from build123d import *

# Parameters (mm, degrees)
F1_DEPTH    = 50.8
F2_W        = 57.15
F2_H        = 38.1
F3_DEPTH    = 6.35
F4_W        = 23.114
F4_H        = 6.604
F4_W_2      = 0.9801145643
F4_H_2      = 5.08
F5_DEPTH    = 2.54
F4_R        = 2.667
F6_DEPTH    = 1.27
F8_DEPTH    = 0.8001
F9_T1_DEPTH = 71.4372925246
F9_T3_DEPTH = 69.6542925277
F11_DEPTH   = 0.8001
F13_DEPTH   = 0.8001
F15_DEPTH   = 0.254
F16_W       = 18.161
F16_H       = 19.05
F17_DEPTH   = 0.8001
F18_DEPTH   = 50.8
F19_W       = 127
F19_H       = 25.4
F20_DEPTH   = 12.7
F21_DEPTH   = 5.08
F22_R       = 1.397
F23_R       = 1.397
F24_DEPTH   = 25.4


# Not quite as in the source:
# - a fillet or chamfer that OpenCascade refuses, or shapes differently, is made with other operations: its cross-section is extruded or revolved along the edge and cut away or added


with BuildPart() as f1:
    # F0 (on Front) → F1 (new body)
    with BuildSketch(Plane.XZ):
        with BuildLine():
            Line((-68.745650351, 20.2095657587), (-68.745650351, 0))
            Line((-68.745650351, 0), (-55.97953596, 0))
            ThreePointArc((-55.97953596, 0), (-44.54953596, 11.43), (-33.11953596, 0))
            Line((-33.11953596, 0), (44.1833575737, 0))
            ThreePointArc((44.1833575737, 0), (55.6133575737, 11.43), (67.0433575737, 0))
            Line((67.0433575737, 0), (83.654349649, 0))
            Line((83.654349649, 0), (83.654349649, 19.05))
            Line((83.654349649, 19.05), (20.154349649, 19.05))
            Line((20.154349649, 19.05), (20.154349649, 50.8))
            Line((20.154349649, 50.8), (-20.485650351, 50.8))
            Line((-20.485650351, 50.8), (-27.103371678, 28.9188353957))
            Line((-27.103371678, 28.9188353957), (-68.745650351, 20.2095657587))
        make_face()
        with BuildLine():
            ThreePointArc((-33.11953596, 0), (-44.54953596, 11.43), (-55.97953596, 0))
            Line((-55.97953596, 0), (-33.11953596, 0))
        make_face()
        with BuildLine():
            ThreePointArc((67.0433575737, 0), (55.6133575737, 11.43), (44.1833575737, 0))
            Line((44.1833575737, 0), (67.0433575737, 0))
        make_face()
    extrude(amount=F1_DEPTH)

    # F2 (on face) → F3 (cut)
    with BuildSketch(Plane.XY.offset(19.05)):
        with Locations((48.729349649, -25.4)):
            Rectangle(F2_W, F2_H)
    extrude(amount=-F3_DEPTH, mode=Mode.SUBTRACT)

    # F4 (on face) → F5 (join)
    with BuildSketch(Plane(origin=(-68.745650351, 0, 0), x_dir=(0, -1, 0), z_dir=(-1, 0, 0))):
        with Locations((25.4, 9.8053713022)):
            Rectangle(F4_W, F4_H)
        Polygon((36.195, 12.3453713022), (36.195, 7.2653713022), (32.6746520766, 7.2653713022), (31.6945375124, 7.2653713022), (29.2964520766, 7.2653713022), (28.3163375124, 7.2653713022), (25.9182520766, 7.2653713022), (24.9381375124, 7.2653713022), (22.5400520766, 7.2653713022), (21.5599375124, 7.2653713022), (19.1618520766, 7.2653713022), (18.1817375124, 7.2653713022), (14.605, 7.2653713022), (14.605, 12.3453713022), (18.1817375124, 12.3453713022), (19.1618520766, 12.3453713022), (21.5599375124, 12.3453713022), (22.5400520766, 12.3453713022), (24.9381375124, 12.3453713022), (25.9182520766, 12.3453713022), (28.3163375124, 12.3453713022), (29.2964520766, 12.3453713022), (31.6945375124, 12.3453713022), (32.6746520766, 12.3453713022), align=None, mode=Mode.SUBTRACT)
        with Locations((18.6717947945, 9.8053713022)):
            Rectangle(F4_W_2, F4_H_2)
        with Locations((22.0499947945, 9.8053713022)):
            Rectangle(F4_W_2, F4_H_2)
        with Locations((25.4281947945, 9.8053713022)):
            Rectangle(F4_W_2, F4_H_2)
        with Locations((28.8063947945, 9.8053713022)):
            Rectangle(F4_W_2, F4_H_2)
        with Locations((32.1845947945, 9.8053713022)):
            Rectangle(F4_W_2, F4_H_2)
    extrude(amount=F5_DEPTH)

    # F4 (on face) → F6 (join)
    with BuildSketch(Plane(origin=(-68.745650351, 0, 0), x_dir=(0, -1, 0), z_dir=(-1, 0, 0))):
        with Locations((6.35, 9.8351975903)):
            Circle(F4_R)
        with Locations((44.45, 9.8351975903)):
            Circle(F4_R)
    extrude(amount=F6_DEPTH)

    # F7 (on face) → F8 (cut)
    with BuildSketch(Plane(origin=(-32.8452255156, 0, 9.9336828416), x_dir=(0, -1, 0), z_dir=(-0.9571813038, 0, 0.2894891219))):
        Polygon((33.562220633, 22.6956736296), (47.9775152107, 22.6956736296), (47.9775152107, 40.2216736296), (2.2575152107, 40.2216736296), (2.2575152107, 22.6956736296), (16.4677330811, 22.6956736296), (15.0759897713, 29.1358400136), (13.6842464615, 33.1220440567), (16.4677330811, 29.1358400136), (17.814220633, 22.6956736296), (32.2157330811, 22.6956736296), (30.8239897713, 29.1358400136), (29.4322464615, 33.1220440567), (32.2157330811, 29.1358400136), align=None)
    extrude(amount=-F8_DEPTH, mode=Mode.SUBTRACT)

    # F9: fillet of radius 5.08 on 2 edges, made by hand

    # F9_s2 → F9_t1 (cut)
    with BuildSketch(Plane.XZ.offset(-10.3186462623)):
        with BuildLine():
            ThreePointArc((-64.7056051643, 21.0545205498), (-67.6083252331, 19.2854983904), (-68.745650351, 16.0821072538))
            Line((-68.745650351, 16.0821072538), (-68.745650351, 20.2095657587))
            Line((-68.745650351, 20.2095657587), (-64.7056051643, 21.0545205498))
        make_face()
    extrude(amount=F9_T1_DEPTH, mode=Mode.SUBTRACT)

    # F9_s4 → F9_t3 (cut)
    with BuildSketch(Plane.XZ.offset(-9.4271462638)):
        with BuildLine():
            ThreePointArc((-21.5772728687, 47.1906047393), (-19.74263992, 49.7990361653), (-16.7147918455, 50.8))
            Line((-16.7147918455, 50.8), (-20.485650351, 50.8))
            Line((-20.485650351, 50.8), (-21.5772728687, 47.1906047393))
        make_face()
    extrude(amount=F9_T3_DEPTH, mode=Mode.SUBTRACT)

    # F10 (on face) → F11 (join)
    with BuildSketch(Plane.XZ.offset(50.8)):
        Polygon((13.9938081476, 45.7206499122), (-16.7147918455, 45.72), (-21.5772728687, 29.6424496777), (-21.5772728687, 5.5124496777), (13.9827271313, 5.5124514391), align=None)
    extrude(amount=F11_DEPTH)

    # F12 (on face) → F13 (join)
    with BuildSketch(Plane(origin=(0, 0, 0), x_dir=(-1, 0, 0), z_dir=(0, 1, 0))):
        Polygon((21.566192252, 29.6467966337), (16.7147918455, 45.72), (-13.993807748, 45.7249966337), (-13.993807748, 5.5167966337), (21.566192252, 5.5167966337), align=None)
    extrude(amount=F13_DEPTH)

    # F14 (on face) → F15 (join)
    with BuildSketch(Plane(origin=(0, 0.8001, 0), x_dir=(-1, 0, 0), z_dir=(0, 1, 0))):
        Polygon((-11.5635488182, 29.6467966337), (18.8161898404, 29.6467966337), (14.9059221148, 43.1567057967), (-11.5635488182, 43.1567057967), align=None)
    extrude(amount=-F15_DEPTH)

    # F16 (on face) → F17 (cut)
    with BuildSketch(Plane.YZ.offset(20.154349649)):
        with Locations((-35.3695, 38.1)):
            Rectangle(F16_W, F16_H)
        with Locations((-15.4305, 38.1)):
            Rectangle(F16_W, F16_H)
    extrude(amount=-F17_DEPTH, mode=Mode.SUBTRACT)

    # F0 (on Front) → F18 (cut)
    with BuildSketch(Plane.XZ):
        with BuildLine():
            ThreePointArc((67.0433575737, 0), (55.6133575737, 11.43), (44.1833575737, 0))
            Line((44.1833575737, 0), (67.0433575737, 0))
        make_face()
        with BuildLine():
            ThreePointArc((-33.11953596, 0), (-44.54953596, 11.43), (-55.97953596, 0))
            Line((-55.97953596, 0), (-33.11953596, 0))
        make_face()
    extrude(amount=F18_DEPTH, mode=Mode.SUBTRACT)

    # F19 (on face) → F20 (join)
    with BuildSketch(Plane(origin=(0, 0, 0), x_dir=(1, 0, 0), z_dir=(0, 0, -1))):
        with Locations((6.3173042834, 25.4)):
            Rectangle(F19_W, F19_H)
    extrude(amount=-F20_DEPTH)

    # F21 (add): a face of the model
    f21_faces = [f1.faces().sort_by_distance(p)[0] for p in [
        (7.7936035623, -25.4, 0),
    ]]
    extrude(f21_faces, amount=F21_DEPTH)

    # F22 (on face) + F23 (on face) → F24 (cut)
    with BuildSketch(Plane(origin=(0, -12.7, 0), x_dir=(-1, 0, 0), z_dir=(0, 1, 0))):
        with Locations((-55.6133575737, 0)):
            Circle(F22_R)
    with BuildSketch(Plane(origin=(0, -12.7, 0), x_dir=(-1, 0, 0), z_dir=(0, 1, 0))):
        with Locations((44.54953596, 0)):
            Circle(F23_R)
    extrude(amount=-F24_DEPTH, mode=Mode.SUBTRACT)


solid = f1.part
Design review of the part built by this model. Coordinates are the model's own, in mm. A direction names the side the tool comes from. Round coordinates to 2 decimals unless told otherwise and drop trailing zeros. Write each loop counter-clockwise with the first axis right and the second up, starting at its lowest first coordinate (ties: lowest second). Pieces come first, ordered by that corner, then holes. Notation, with made-up numbers: (33.25, 24.25) -> (76.25, 24.25) arc R30 ccw to (76.25, 55.25) -> close; hole circle Ø10 at (35.5, 77.25). An arc over 180 degrees is marked (long way). One line per item, written item: value. Start each with the question number.
Q1. Add section A-A (x = -41). Give the boundary of the cut face in (y, z), then the cut area to 3 significant figures.
Q2. To check wall thickness, follow probe 1 along X at (y, z) = (-28.5, 1); probe 2 along X at (y, z) = (-8.5, 6); probe 3 along Z at (x, y) = (62.5, -20). State the ranges of each line that lie inside material, in increasing order.
Q3. Insertion check: P1, Ø5, axis at y = -11.5, z = 23, coming from the -X side; P2, Ø1.5, axis at x = 50, y = -28, coming from the +Z side; P3, Ø5, axis at x = -46, z = 0, coming from the -Y side. Each pin has a flat end and moves straight along its axis. Give the tip position at first contact, or say it passes through.
Q4. Tool access review of faces 5 (the face through (48, -6.35, 16)), 6 (the face through (-43.154, -25.222, 0.061)), 7 (the face through (-33.12, -6, -3)), 8 (the face through (-45, -38.1, 3)), 9 (the face through (-69.37, -7.58, 7.47)): name each direction out of +Z, -Z, +X, -X, +Y, -Y from which nothing blocks a thin tool from reaching the whole face with its end or side.
Q5. The part is to be moulded in two halves that separate along X. For faces 1 (the face through (20.154, -25, 31)), 2 (the face through (-19.174, 0.394, 37.571)), 3 (the face through (-55.98, -6, -3)), 4 (the face through (6, 0, 5)), say which applies: pulls with the +X half, pulls with the -X half, needs draft (parallel to the pull), parting line crosses it, or undercut.
Response:
1. outline: (-50.8, 10.86) -> (-38.1, 10.86) -> (-38.1, -5.08) -> (-12.7, -5.08) -> (-12.7, 10.86) -> (0, 10.86) -> (0, 26.01) -> (-50.8, 26.01) -> close
1. area: 1,170 mm^2
2. probe 1: x = -68.75 to -45.53, -43.57 to 54.64, 56.59 to 83.65
2. probe 2: x = -68.75 to -54.28, -34.82 to 45.88, 65.34 to 83.65
2. probe 3: z = -5.08 to 12.7
3. P1: stops at x = -66.17
3. P2: stops at z = 12.7
3. P3: stops at y = -38.1
4. face 5: +Z
4. face 6: +Y, -Y
4. face 7: -Z, +Y
4. face 8: -Z, -Y
4. face 9: -X
5. face 1: undercut
5. face 2: pulls with the -X half
5. face 3: undercut
5. face 4: needs draft
